Here's the drawing with two shaded views (mm, measured from the low corner). I have some questions. A direction names the side the tool comes from. Round coordinates to 2 decimals unless told otherwise and drop trailing zeros. Loops run counter-clockwise (first coordinate to the right, second up) from the corner with the lowest first, then second, coordinate; pieces in that order, holes last. Notation, with made-up numbers: M 86.25,39 L 128.25,39 A18 ccw 128.25,50 Z; hole C -15.75,-40 d9. An arc over 180 degrees is marked long. Answer as a JSON object with one key per item and string values.
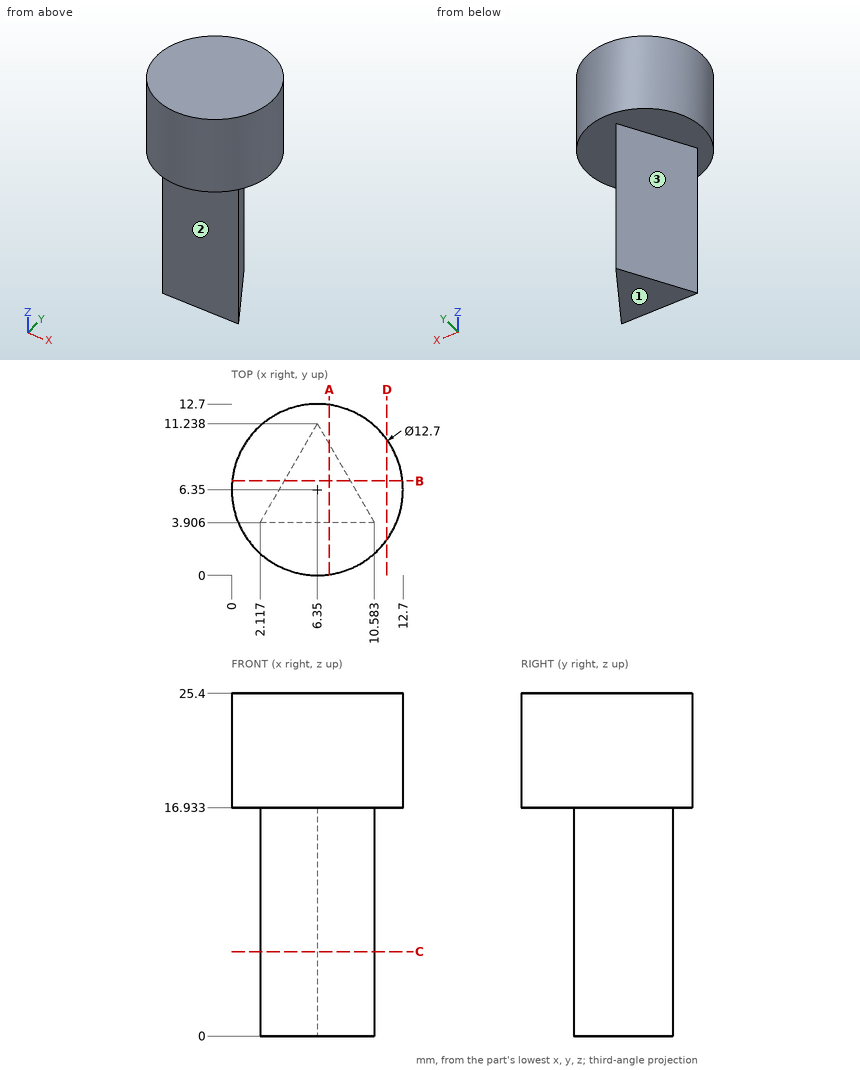
Item 1: For P1, Ø2.5, axis at x = 5.5, z = 8.5, coming from the -Y side; P2, Ø6, axis at y = 1.5, z = 21, coming from the +X side (1 decimal), each with a flat end and sliding along its axis, tell me the tip position at first contact or that it passes through.
Solution:
{"P1": "stops at y = 3.91", "P2": "stops at x = 12.4"}
Item 2: I want a section at A-A on x = 7.25. List the corners of the cut face in (y, z) for me.
Solution:
{"outline": "M 0.06,16.93 L 3.91,16.93 L 3.91,0 L 9.68,0 L 9.68,16.93 L 12.64,16.93 L 12.64,25.4 L 0.06,25.4 Z"}
Item 3: I want a section at B-B on y = 7. List the corners of the cut face in (x, z) for me.
Solution:
{"outline": "M 0.03,16.93 L 3.9,16.93 L 3.9,0 L 8.8,0 L 8.8,16.93 L 12.67,16.93 L 12.67,25.4 L 0.03,25.4 Z"}
Item 4: I want a section at D-D on x = 11.5. List the corners of the cut face in (y, z) for me (1 decimal).
Solution:
{"outline": "M 2.6,16.9 L 10.1,16.9 L 10.1,25.4 L 2.6,25.4 Z"}
Item 5: I want a section at C-C on z = 6.25. List the corners of the cut face in (x, y) for me.
Solution:
{"outline": "M 2.12,3.91 L 10.58,3.91 L 6.35,11.24 Z"}
Item 6: For the marked faces 1, 2 and 3, which set-ups out of +Z, -Z, +X, -X, +Y, -Y let a thin tool reach every point of the face, with its end or its side?
Solution:
{"face 1": "-Z, +X, -X, +Y, -Y", "face 2": "-Z, +X, -X, -Y", "face 3": "-Z, -X, +Y"}
Item 7: If I drill on L1, parallel to Z at x = 4, y = 1; L2, parallel to Y at x = 7.5, z = 18 (1 decimal); L3, parallel to X at y = 2.75, z = 22, over which ranges is the centre line in solid material (lowest first)? Write a range as from..to.
Solution:
{"L1": "z = 16.93..25.4", "L2": "y = 0.1..12.6", "L3": "x = 1.12..11.58"}
